from build123d import *

# Parameters (mm, degrees)
SKETCH1_W           = 23.15
SKETCH1_H           = 11.82
BOSS_EXTRUDE1_DEPTH = 22.2
SKETCH2_W           = 31.87
SKETCH2_H           = 11.82
BOSS_EXTRUDE2_DEPTH = 1.55
SKETCH3_R           = 1
CUT_EXTRUDE1_DEPTH  = 7.7
CUT_EXTRUDE2_DEPTH  = 12.82
SKETCH5_R           = 5.91
BOSS_EXTRUDE3_DEPTH = 4
SKETCH6_R           = 2.375
BOSS_EXTRUDE4_DEPTH = 2.75
SKETCH7_R           = 0.375
CUT_EXTRUDE3_DEPTH  = 2.75


with BuildPart() as part:
    # Sketch1 → Boss-Extrude1 (new body)
    with BuildSketch(Plane(origin=(0, 0, 0), x_dir=(1, 0, 0), z_dir=(0, 1, 0))):
        with Locations((11.575, 5.91)):
            Rectangle(SKETCH1_W, SKETCH1_H)
    extrude(amount=BOSS_EXTRUDE1_DEPTH)

    # Sketch2 → Boss-Extrude2 (add)
    with BuildSketch(Plane(origin=(0, 15.5, 0), x_dir=(-1, 0, 0), z_dir=(0, 1, 0))):
        with Locations((-11.575, -5.91)):
            Rectangle(SKETCH2_W, SKETCH2_H)
    extrude(amount=BOSS_EXTRUDE2_DEPTH)

    # Sketch3 → Cut-Extrude1 (cut, through all)
    with BuildSketch(Plane(origin=(0, 15.5, 0), x_dir=(-1, 0, 0), z_dir=(0, 1, 0))):
        with Locations((-25.33, -5.91)):
            Circle(SKETCH3_R)
        with Locations((2.18, -5.91)):
            Circle(SKETCH3_R)
    extrude(amount=CUT_EXTRUDE1_DEPTH, mode=Mode.SUBTRACT)

    # Sketch4 → Cut-Extrude2 (cut, through all)
    with BuildSketch(Plane.XY):
        Polygon((-3.075644921, 5.946535733), (9.026256409, -3.679976689), (-2.538069932, -3.679976689), align=None)
    extrude(amount=-CUT_EXTRUDE2_DEPTH, mode=Mode.SUBTRACT)

    # Sketch5 → Boss-Extrude3 (add)
    with BuildSketch(Plane(origin=(0, 22.2, 0), x_dir=(1, 0, 0), z_dir=(0, 1, 0))):
        with Locations((17.24, 5.91)):
            Circle(SKETCH5_R)
    extrude(amount=BOSS_EXTRUDE3_DEPTH)

    # Sketch6 → Boss-Extrude4 (add)
    with BuildSketch(Plane(origin=(0, 26.2, 0), x_dir=(1, 0, 0), z_dir=(0, 1, 0))):
        with Locations((17.24, 5.91)):
            Circle(SKETCH6_R)
    extrude(amount=BOSS_EXTRUDE4_DEPTH)

    # Sketch7 → Cut-Extrude3 (cut)
    with BuildSketch(Plane(origin=(0, 28.95, 0), x_dir=(1, 0, 0), z_dir=(0, 1, 0))):
        with Locations((17.24, 5.91)):
            Circle(SKETCH7_R)
    extrude(amount=-CUT_EXTRUDE3_DEPTH, mode=Mode.SUBTRACT)


solid = part.part
Work out the finished part from the listing and answer in its coordinate system (mm). A direction names the side the tool comes from. Coordinates: 2 decimals unless noted, no trailing zeros. Loops run counter-clockwise (first coordinate to the right, second up) from the corner with the lowest first, then second, coordinate; pieces in that order, holes last. Notation, with made-up numbers: M 8.25,-3 L 39.25,-3 A7 cw 39.25,4 Z; hole C -35.75,54.25 d10. An arc over 180 degrees is marked long. Answer in a Markdown table with one row per item. Add a question column.
1. Find section D-D, the plane x = 18.5. Write down the section's boundary in (y, z), then the cut area to 3 significant figures.
2. The mould has two halves that part along Z. Classify faces 1 (the cylindrical face through (22.877, 24.172, -7.685)), 2 (the cylindrical face through (-3.134, 16.264, -5.61)), 3 (the flat face through (2.169, 1.775, -5.827)): pulls with the +Z half, pulls with the -Z half, needs draft (parallel to the pull), parting line crosses it, or undercut.
3. Consider L1, parallel to X at y = 15.95, z = -5.91; L2, parallel to Z at x = 17.24, y = 27.95 (3 decimals); L3, parallel to X at y = 27.9, z = -5.91 (3 decimals). Determine where each line is inside the solid, lowest interval first.
4. Find section C-C, the plane z = -4.5. Write down the section's boundary in (x, y), then the cut area to 3 significant figures.
5. Find section A-A, the plane x = 25.33. Write down the section's boundary in (y, z), then the cut area to 3 significant figures.
6. A tool of negligible diameter and unlimited length cuts with its end or side. For faces 4 (the flat face through (23.15, 20, -6)), 5 (the flat face through (0, 9, -6)), 6 (the flat face through (0, 20, -6)), 7 (the flat face through (17, 26.2, -3)), from which of +Z, -Z, +X, -X, +Y, -Y can it reach the whole face along a straight path? Write none if from no direction.
7. Flat-ended cylindrical pins translate along their axes: P1, Ø3, axis at x = 19, z = -3, coming from the +Y side; P2, Ø1.3, axis at x = -1.5, z = -3, coming from the -Y side; P3, Ø3, axis at x = -2.18, z = -5.91, coming from the +Y side; P4, Ø6, axis at x = 8, z = -5.5, coming from the +Y side. Find the tip coordinate at first contact, or state that the pin passes through.
8. Find section B-B, the plane y = 24.25. Write down the section's boundary in (x, z), then the cut area to 3 significant figures.
Reported:
| question | item | result |
|---|---|---|
| 1 | outline | M 0,-11.82 L 22.2,-11.82 L 22.2,-11.68 L 26.2,-11.68 L 26.2,-7.92 L 28.95,-7.92 L 28.95,-3.9 L 26.2,-3.9 L 26.2,-0.14 L 22.2,-0.14 L 22.2,0 L 0,0 Z |
| 1 | area | 320 mm^2 |
| 2 | face 1 | parting line crosses it |
| 2 | face 2 | undercut |
| 2 | face 3 | needs draft |
| 3 | L1 | x = -4.36 to -3.18, -1.18 to 24.33, 26.33 to 27.51 |
| 3 | L2 | z = -8.285 to -6.285, -5.535 to -3.535 |
| 3 | L3 | x = 14.865 to 16.865, 17.615 to 19.615 |
| 4 | outline | M -4.36,15.5 L 0,15.5 L 0,3.5 L 4.4,0 L 23.15,0 L 23.15,15.5 L 27.51,15.5 L 27.51,17.05 L 23.15,17.05 L 23.15,22.2 L 22.98,22.2 L 22.98,26.2 L 19.15,26.2 L 19.15,28.95 L 15.33,28.95 L 15.33,26.2 L 11.5,26.2 L 11.5,22.2 L 0,22.2 L 0,17.05 L -4.36,17.05 Z |
| 4 | area | 576 mm^2 |
| 5 | outline | M 15.5,-11.82 L 17.05,-11.82 L 17.05,-6.91 L 15.5,-6.91 Z; M 15.5,-4.91 L 17.05,-4.91 L 17.05,0 L 15.5,0 Z |
| 5 | area | 15.2 mm^2 |
| 6 | face 4 | +Z, -Z, +X, +Y |
| 6 | face 5 | +Z, -Z, -X, -Y |
| 6 | face 6 | +Z, -Z, -X, +Y |
| 6 | face 7 | +Y |
| 7 | P1 | stops at y = 28.95 |
| 7 | P2 | stops at y = 15.5 |
| 7 | P3 | stops at y = 17.05 |
| 7 | P4 | stops at y = 22.2 |
| 8 | outline | C 17.24,-5.91 d11.82 |
| 8 | area | 110 mm^2 |
